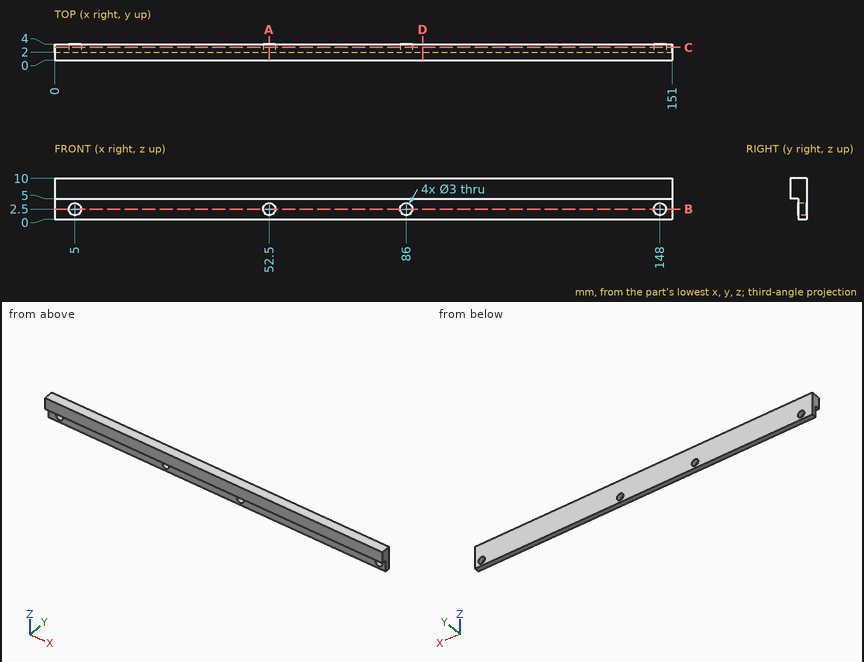
Source: three-view drawing plus pictorial views. Frame: mm from the lowest corner of the part. Coordinates: 2 decimals unless noted, no trailing zeros. Order: outer loops, then holes, each group sorted by start corner. A loop starts at its lowest first (then second) coordinate and runs counter-clockwise, first axis right, second up. Notation, with made-up numbers: M 67,86 L 86,86 A15 cw 86,103 Z; hole C 72.5,-31 d5. An arc over 180 degrees is marked long. Answer in a Markdown table with one row per item.
(1) Material intervals for line 1 (X direction, y = 2.5, z = 2.5); line 2 (Z direction, x = 148, y = 2.9); line 3 (X direction, y = 3.3, z = 3), sorted ascending. Write a range as [from, to].
Numbers:
| item | result |
|---|---|
| line 1 | x = [0, 3.5], [6.5, 51], [54, 84.5], [87.5, 146.5], [149.5, 151] |
| line 2 | z = [0, 1], [4, 10] |
| line 3 | x = [0, 3.59], [6.41, 51.09], [53.91, 84.59], [87.41, 146.59], [149.41, 151] |
(2) Section query B-B, the plane z = 2.5. Output: boundary loops of the cut face in (x, y).
Numbers:
| item | result |
|---|---|
| outline | M 0,2 L 3.5,2 L 3.5,4 L 0,4 Z; M 6.5,2 L 51,2 L 51,4 L 6.5,4 Z; M 54,2 L 84.5,2 L 84.5,4 L 54,4 Z; M 87.5,2 L 146.5,2 L 146.5,4 L 87.5,4 Z; M 149.5,2 L 151,2 L 151,4 L 149.5,4 Z |
(3) Section query A-A, the plane x = 52.5. Output: boundary loops of the cut face in (y, z).
Numbers:
| item | result |
|---|---|
| outline | M 0,5 L 2,5 L 2,4 L 4,4 L 4,10 L 0,10 Z; M 2,0 L 4,0 L 4,1 L 2,1 Z |
(4) Section query D-D, the plane x = 90. Output: boundary loops of the cut face in (y, z), plus the area to 3 significant figures.
Numbers:
| item | result |
|---|---|
| outline | M 0,5 L 2,5 L 2,0 L 4,0 L 4,10 L 0,10 Z |
| area | 30.0 mm^2 |
(5) Section query C-C, the plane y = 3.15. Output: boundary loops of the cut face in (x, z).
Numbers:
| item | result |
|---|---|
| outline | M 0,0 L 151,0 L 151,10 L 0,10 Z; hole C 5,2.5 d3; hole C 52.5,2.5 d3; hole C 86,2.5 d3; hole C 148,2.5 d3 |
(6) Contact query for flat-ended pins moving along their axis: pin 1 Ø4 at (x, z) = (68, 2.5) entering from -Y; pin 2 Ø1.6 at (x, y) = (80, 1) entering from -Z. Output: stop coordinate, or through.
Numbers:
| item | result |
|---|---|
| pin 1 | stops at y = 2 |
| pin 2 | stops at z = 5 |
